Autodesk Inventor part; units mm, degrees
ref_plane "YZ Plane" through (0, 0, 0) normal (1, 0, 0) x (0, 1, 0)
ref_plane "XZ Plane" through (0, 0, 0) normal (0, 1, 0) x (-1, 0, 0)
ref_plane "XY Plane" through (0, 0, 0) normal (0, 0, 1) x (1, 0, 0)
sketch "Sketch1" plane through (0, 0, 0) normal (0, 1, 0) x (-1, 0, 0)
  circle A0 centre (0, 0) radius 6.35
  circle A1 centre (0, 0) radius 4
  line L0 (-1.5875, 6.1484) -> (-1.5875, 4.7625)
  line L1 (-1.5875, 4.7625) -> (1.5875, 4.7625)
  line L2 (1.5875, 4.7625) -> (1.5875, 6.1484)
  line L3 (0, 6.35) -> (0, 0) construction
  line L4 (0, 0) -> (4.4901, -4.4901) construction
  line L5 (0, 0) -> (6.35, 0) construction
  line L6 (2.0315, -3.4457) -> (2.8284, -4.2426)
  line L7 (2.8284, -4.2426) -> (4.2426, -2.8284)
  line L8 (4.2426, -2.8284) -> (3.4457, -2.0315)
  line L9 (2.8284, -2.8284) -> (3.5355, -3.5355) construction
  point P0 (0, 4.7625)
  dimension "d0" = 12.7
  dimension "d1" = 8
  dimension "d4" = 3.175
  dimension "d5" = 45
  dimension "d6" = 2
  dimension "d8" = 1.5875
  dimension "d9" = 1
extrude "Extrusion1" add sketch "Sketch1" along normal blind 19.05 contours A0 L0 L1 L2 picked at (1.2402, -5.3906)
chamfer "Chamfer1" distance 0.254 angle 45 2 edges at (0, 19.05, -6.35) (0, 0, -6.35)
properties part number "0.5 inch Shaft to 8mm Shaft Insert" material "Aluminum 6061"
Here's how the part is built. I have some questions about the finished solid (model axes, mm). A direction names the side the tool comes from. Round coordinates to 2 decimals unless told otherwise and drop trailing zeros. Loops run counter-clockwise (first coordinate to the right, second up) from the corner with the lowest first, then second, coordinate; pieces in that order, holes last. Notation, with made-up numbers: (83, 1) -> (127, 1) arc R37 cw to (127, 39) -> close; hole circle Ø5 at (41, -6.5). An arc over 180 degrees is marked (long way). Write each question's results on one line, items separated by ' | '.
(1) We'd pull the mould along Z, two halves only. Please class faces 1 (the face through (-3.526, 9.392, -3.545)), 2 (the face through (-0.25, 18.92, -6.22)), 3 (the face through (1.4, 19.05, -4)): released by +Z, released by -Z, zero draft, split by the parting line, or undercut.
Worked answers:
face 1: undercut | face 2: split by the parting line | face 3: zero draft
(2) If we section it at A-A, the plane x = 0: List the corners of the cut face in (y, z) for me, then the cut area to 3 significant figures.
Worked answers:
outline: (0, -6.1) -> (0.25, -6.35) -> (18.8, -6.35) -> (19.05, -6.1) -> (19.05, -4) -> (0, -4) -> close; (0, 4) -> (19.05, 4) -> (19.05, 4.76) -> (0, 4.76) -> close | area: 59.2 mm2
(3) If I drill on L1, parallel to X at y = 9.75, z = 0; L2, parallel to Z at x = 0, y = 14; L3, parallel to Z at x = 0.75, y = 6.75, over which ranges is the centre line in solid material (lowest first)?
Worked answers:
L1: -6.35 to -4, 4 to 6.35 | L2: -6.35 to -4, 4 to 4.76 | L3: -6.31 to -3.93, 3.93 to 4.76
(4) For P1, Ø1.1, axis at y = 14, z = 5, coming from the -X side; P2, Ø3, axis at y = 11.5, z = 3.5, coming from the +X side; P3, Ø1.6, axis at x = 0.5, y = 10.5, coming from the +Z side; P4, Ø5, axis at x = -2, y = 7.5, coming from the -Z side, each with a flat end and sliding along its axis, tell me the tip position at first contact or that it passes through.
Worked answers:
P1: x = -4.53 | P2: x = 6.03 | P3: z = 4.76 | P4: z = -6.35
(5) For faces 4 (the face through (0, 9, 4.762)), 5 (the face through (-0.257, 9.395, -6.345)), which set-ups out of +Z, -Z, +X, -X, +Y, -Y let a thin tool reach every point of the face, with its end or its side?
Worked answers:
face 4: +Z, +Y, -Y | face 5: +Y, -Y
(6) If we section it at B-B, the plane y = 5: List the corners of the cut face in (x, z) for me.
Worked answers:
outline: (-1.59, 4.76) -> (-1.59, 6.15) arc R6.35 ccw (long way) to (1.59, 6.15) -> (1.59, 4.76) -> close; hole (-4.24, -2.83) -> (-2.83, -4.24) -> (-2.03, -3.45) arc R4 ccw (long way) to (-3.45, -2.03) -> close
